from build123d import *

# Parameters (mm, degrees)
F1_DEPTH = 10
F3_DEPTH = 8.001
F4_DEPTH = 10


with BuildPart() as f1:
    # F0 (on Front) → F1 (new body)
    with BuildSketch(Plane.XZ):
        Polygon((2, 8), (0, 8), (0, 0), (10, 0), (10, 2), align=None)
    extrude(amount=-F1_DEPTH)

    # F2 (on face) → F3 (cut, through all)
    with BuildSketch(Plane(origin=(0, 0, 0), x_dir=(1, 0, 0), z_dir=(0, 0, -1))):
        Polygon((10, 0), (4, 0), (10, -6), align=None)
    extrude(amount=-F3_DEPTH, mode=Mode.SUBTRACT)

    # F2 (on face) → F4 (join)
    with BuildSketch(Plane(origin=(0, 0, 0), x_dir=(1, 0, 0), z_dir=(0, 0, -1))):
        Polygon((5, -6), (0, -1), (0, -10), (5, -10), align=None)
    extrude(amount=-F4_DEPTH)


solid = f1.part
Build history of the part. All positions in model axes, mm. A direction names the side the tool comes from. Round coordinates to 2 decimals unless told otherwise and drop trailing zeros. Order: outer loops, then holes, each group sorted by start corner. A loop starts at its lowest first (then second) coordinate and runs counter-clockwise, first axis right, second up. Notation, with made-up numbers: M 67.25,45 L 102.25,45 A23 ccw 102.25,84 Z; hole C 67.25,12 d1. An arc over 180 degrees is marked long. Use CSV: the item, a comma, the result in double quotes. Start each with the question number.
(1) Tool access for faces 1 (the face through (6, 5, 5)), 2 (the face through (5, 8, 8)), 3 (the face through (6, 2, 2)): list every direction of +Z, -Z, +X, -X, +Y, -Y with a clear straight run to the whole face (end or side of a thin tool).
(2) Drill centre lines: probe 1 along Y at (x, z) = (7, 3.25); probe 2 along Y at (x, z) = (6, 4); probe 3 along X at (y, z) = (1.5, 7.25). Where is each one in solid material? Low to high.
(3) Cut at B-B on z = 3.5. List the corners of the cut face in (x, y).
(4) Cut at D-D on y = 7.75. List the corners of the cut face in (x, z).
(5) Flat gauge pin, fed straight in: P1, Ø2, axis at y = 9, z = 8, coming from the +X side. Where does the tip first touch, or does it go through?
(6) Cut at A-A on y = 5. List the corners of the cut face in (x, z), then the cut area to 3 significant figures.
(7) Cut at C-C on x = 7.75. List the corners of the cut face in (y, z).
Findings:
1,face 1,"+Z, +X, -Y"
1,face 2,"+Z, +X, +Y, -Y"
1,face 3,"+Z, -Z, +X, -Y"
2,probe 1,"y = 3 to 10"
2,probe 2,"y = 2 to 10"
2,probe 3,"x = 0 to 3"
3,outline,"M 0,0 L 4,0 L 8,4 L 8,10 L 0,10 Z"
4,outline,"M 0,0 L 10,0 L 10,2 L 5,5.75 L 5,10 L 0,10 Z"
5,P1,"stops at x = 5"
6,outline,"M 0,0 L 9,0 L 9,2.75 L 4,6.5 L 4,10 L 0,10 Z"
6,area,"63.1 mm^2"
7,outline,"M 3.75,0 L 10,0 L 10,3.69 L 3.75,3.69 Z"
